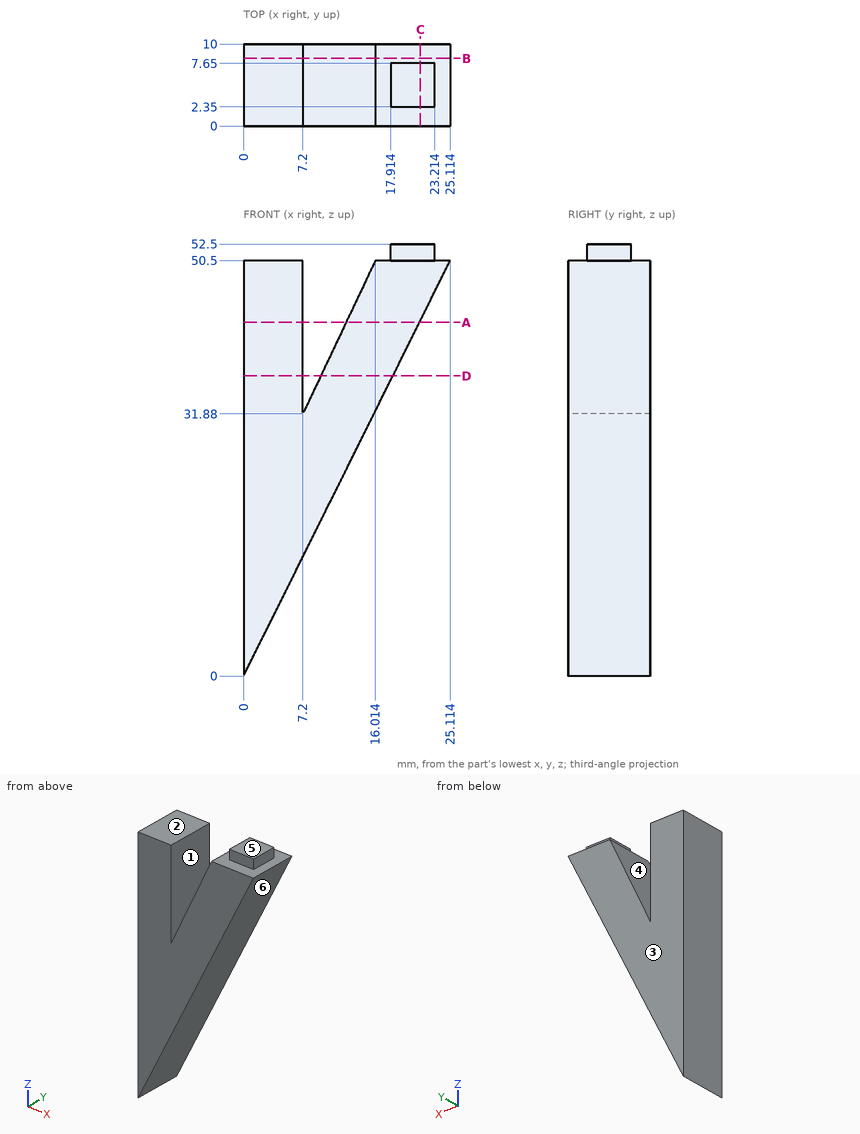
Design review of the part shown in the three views and the two pictorial views. Dimensions are in mm from the part's minimum x, y and z. A direction names the side the tool comes from. Round coordinates to 2 decimals unless told otherwise and drop trailing zeros. Order: outer loops, then holes, each group sorted by start corner. A loop starts at its lowest first (then second) coordinate and runs counter-clockwise, first axis right, second up. Notation, with made-up numbers: M -21,8 L 23,8 A17 cw 23,23 Z; hole C 69,6.25 d5. An arc over 180 degrees is marked long. Put each result on its own line as item: value.
Q1. Consider section D-D (z = 36.5). State the section outline as (x, y) points, and give its area (3 significant figures).
Reported:
outline: M 0,0 L 7.2,0 L 7.2,10 L 0,10 Z; M 9.39,0 L 18.15,0 L 18.15,10 L 9.39,10 Z
area: 160 mm²
Q2. Consider section C-C (x = 21.5). State the section outline as (y, z) points, and give its area (3 significant figures).
Reported:
outline: M 0,43.23 L 10,43.23 L 10,50.5 L 7.65,50.5 L 7.65,52.5 L 2.35,52.5 L 2.35,50.5 L 0,50.5 Z
area: 83.3 mm²
Q3. Consider section A-A (z = 43). State the section outline as (x, y) points.
Reported:
outline: M 0,0 L 7.2,0 L 7.2,10 L 0,10 Z; M 12.46,0 L 21.38,0 L 21.38,10 L 12.46,10 Z
Q4. Insertion check: pin 1 Ø2 at (y, z) = (2.5, 41.5) entering from +X; pin 2 Ø1 at (y, z) = (3, 25) entering from +X; pin 3 Ø1 at (x, z) = (21.5, 51.5) entering from -Y. Each pin has a flat end and moves straight along its axis. Give the tip position at first contact, or say it passes through.
Reported:
pin 1: x = 21.14
pin 2: x = 12.68
pin 3: y = 2.35
Q5. To check wall thickness, follow line 1 (X direction, y = 3.25, z = 35); line 2 (X direction, y = 3.75, z = 47); line 3 (Z direction, x = 12, y = 2.5). State the ranges of each line that lie inside material, in increasing order.
Reported:
line 1: 0 to 7.2, 8.68 to 17.41
line 2: 0 to 7.2, 14.36 to 23.37
line 3: 24.13 to 42.02
Q6. Consider section B-B (y = 8.25). State the section outline as (x, z) points.
Reported:
outline: M 0,0 L 25.11,50.5 L 16.01,50.5 L 7.2,31.88 L 7.2,50.5 L 0,50.5 Z
Q7. Draft analysis for pull direction X (two halves, no side actions). For the marked faces 4, 5 and 6, state which applies: released by +X, released by -X, zero draft, split by the parting line, or undercut.
Reported:
face 4: undercut
face 5: zero draft
face 6: released by +X
Q8. Machinability: for the marked faces 1, 2 and 3, which of the approach directions +Z, -Z, +X, -X, +Y, -Y give a long, thin tool a straight path to every point of the face, cutting with its end or side? Answer none if there is none.
Reported:
face 1: +Z, +Y, -Y
face 2: +Z, -X, +Y, -Y
face 3: +Z, -Z, +X, -X, +Y
